Here's how the part is built. I have some questions about the finished solid (model axes, mm). A direction names the side the tool comes from. Coordinates: 2 decimals unless noted, no trailing zeros. Write each loop counter-clockwise with the first axis right and the second up, starting at its lowest first coordinate (ties: lowest second). Pieces come first, ordered by that corner, then holes. Notation, with made-up numbers: (43.5, -33.5) -> (57.5, -33.5) arc R21 cw to (57.5, -26.5) -> close; hole circle Ø3 at (65, -37). An arc over 180 degrees is marked (long way). Put each result on its own line as item: value.
```python
from build123d import *

# Parameters (mm, degrees)
CROQUIS1_R                = 20
SALIENTE_EXTRUIR1_DEPTH   = 45
SALIENTE_EXTRUIR1_2_DEPTH = 45
CROQUIS2_W                = 40
CROQUIS2_H                = 80
SALIENTE_EXTRUIR2_DEPTH   = 45
CORTAR_EXTRUIR2_DEPTH     = 7.6
CROQUIS4_R                = 5.5
CORTAR_EXTRUIR3_DEPTH     = 50
CROQUIS5_W                = 20
CROQUIS5_H                = 40
CORTAR_EXTRUIR4_DEPTH     = 40
CROQUIS6_W                = 20
CROQUIS6_H                = 6.5
CROQUIS6_H_2              = 7
CORTAR_EXTRUIR5_DEPTH     = 12
CORTAR_EXTRUIR6_START     = -27
CROQUIS7_W                = 20
CROQUIS7_H                = 13.910937509
CORTAR_EXTRUIR6_DEPTH     = 12


with BuildPart() as part:
    # Croquis1 → Saliente-Extruir1 (new body)
    with BuildSketch(Plane(origin=(0, 0, 0), x_dir=(0, 1, 0), z_dir=(0, 0, 1))):
        with Locations(Location((-40, 0, 0), (0, 0, 90))):
            Circle(CROQUIS1_R)
    extrude(amount=SALIENTE_EXTRUIR1_DEPTH)



with BuildPart() as body_2:
    # Croquis1 → Saliente-Extruir1 2 (new body)
    with BuildSketch(Plane(origin=(0, 0, 0), x_dir=(0, 1, 0), z_dir=(0, 0, 1))):
        with Locations(Location((40, 0, 0), (0, 0, 90))):
            Circle(CROQUIS1_R)
    extrude(amount=SALIENTE_EXTRUIR1_2_DEPTH)


with BuildPart() as part_1:
    add(part.part)

    add(body_2.part)  # Saliente-Extruir2 merges body 2
    # Croquis2 → Saliente-Extruir2 (add)
    with BuildSketch(Plane.XY.offset(45)):
        Rectangle(CROQUIS2_W, CROQUIS2_H)
    extrude(amount=-SALIENTE_EXTRUIR2_DEPTH)

    # Croquis3 → Cortar-Extruir2 (cut)
    with BuildSketch(Plane.XY.offset(45)):
        with BuildLine():
            Line((-16.5, 42.5), (-4.355962306, 43.357914886))
            Line((-4.355962306, 43.357914886), (-2.5, 56.5))
            ThreePointArc((-2.5, 56.5), (0, 59), (2.5, 56.5))
            Line((2.5, 56.5), (3.889087297, 43.889087297))
            Line((3.889087297, 43.889087297), (16.5, 42.5))
            ThreePointArc((16.5, 42.5), (19, 40), (16.5, 37.5))
            Line((16.5, 37.5), (3.889087297, 36.110912703))
            Line((3.889087297, 36.110912703), (2.5, 23.5))
            ThreePointArc((2.5, 23.5), (0, 21), (-2.5, 23.5))
            Line((-2.5, 23.5), (-3.889087297, 36.110912703))
            Line((-3.889087297, 36.110912703), (-16.5, 37.5))
            ThreePointArc((-16.5, 37.5), (-19, 40), (-16.5, 42.5))
        make_face()
    extrude(amount=-CORTAR_EXTRUIR2_DEPTH, mode=Mode.SUBTRACT)

    # Croquis4 → Cortar-Extruir3 (cut)
    with BuildSketch(Plane.XY.offset(45)):
        with Locations((0, 40)):
            Circle(CROQUIS4_R)
    extrude(amount=-CORTAR_EXTRUIR3_DEPTH, mode=Mode.SUBTRACT)

    # Croquis5 → Cortar-Extruir4 (cut)
    with BuildSketch(Plane(origin=(0, 0, 0), x_dir=(1, 0, 0), z_dir=(0, 0, -1))):
        with Locations((0, 30)):
            Rectangle(CROQUIS5_W, CROQUIS5_H)
    extrude(amount=-CORTAR_EXTRUIR4_DEPTH, mode=Mode.SUBTRACT)

    # Croquis6 → Cortar-Extruir5 (cut)
    with BuildSketch(Plane(origin=(0, 0, 0), x_dir=(1, 0, 0), z_dir=(0, 0, -1))):
        with Locations((0, 53.25)):
            Rectangle(CROQUIS6_W, CROQUIS6_H)
        with Locations((0, 6.5)):
            Rectangle(CROQUIS6_W, CROQUIS6_H_2)
    extrude(amount=-CORTAR_EXTRUIR5_DEPTH, mode=Mode.SUBTRACT)

    # Croquis7 → Cortar-Extruir6 (cut)
    with BuildSketch(Plane(origin=(0, 0, 0), x_dir=(1, 0, 0), z_dir=(0, 0, -1)).offset(CORTAR_EXTRUIR6_START)):
        with Locations((0, 56.955468755)):
            Rectangle(CROQUIS7_W, CROQUIS7_H)
    extrude(amount=-CORTAR_EXTRUIR6_DEPTH, mode=Mode.SUBTRACT)


solid = part_1.part
```
Item 1: Imagine slicing it at C-C on z = 30.5. Write out the boundary of the cut face in (x, y), then the cut area to 3 significant figures.
Output:
outline: (-20, -40) arc R20 ccw to (-10, -57.32) -> (-10, -10) -> (10, -10) -> (10, -57.32) arc R20 ccw to (20, -40) -> (20, 40) arc R20 ccw to (-20, 40) -> close; hole circle Ø11 at (0, 40)
area: 3,380 mm²
Item 2: For P1, Ø10, axis at x = 4.5, y = -33.5, coming from the -Z side; P2, Ø2, axis at x = 3.5, y = -10.5, coming from the -Z side; P3, Ø4, axis at x = 11, z = 16, coming from the +Y side, each with a flat end and sliding along its axis, tell me the tip position at first contact or that it passes through.
Output:
P1: stops at z = 40
P2: stops at z = 12
P3: stops at y = 57.86
Item 3: Imagine slicing it at A-A on x = 0. Write out the boundary of the cut face in (y, z).
Output:
outline: (-60, 0) -> (-56.5, 0) -> (-56.5, 12) -> (-50, 12) -> (-50, 27) -> (-60, 27) -> close; (-60, 39) -> (-50, 39) -> (-50, 40) -> (-10, 40) -> (-10, 12) -> (-3, 12) -> (-3, 0) -> (34.5, 0) -> (34.5, 37.4) -> (21, 37.4) -> (21, 45) -> (-60, 45) -> close; (45.5, 0) -> (60, 0) -> (60, 45) -> (59, 45) -> (59, 37.4) -> (45.5, 37.4) -> close
Item 4: If we mould it in two halves opening along Z, with no side actions, what happens to faces 5 (the flat face through (0, -10, 26)), 6 (the flat face through (-11, 40, 37.4)), 7 (the flat face through (0, 14, 0)), 8 (the flat face through (0, -55, 39))? For each: released by +Z, released by -Z, zero draft, split by the parting line, or undercut.
Output:
face 5: zero draft
face 6: released by +Z
face 7: released by -Z
face 8: undercut
Item 5: Imagine slicing it at B-B on z = 4.5. Write out the boundary of the cut face in (x, y), then the cut area to 3 significant figures.
Output:
outline: (-20, -40) arc R20 ccw to (20, -40) -> (20, 40) arc R20 ccw to (-20, 40) -> close; hole (-10, -56.5) -> (10, -56.5) -> (10, -3) -> (-10, -3) -> close; hole circle Ø11 at (0, 40)
area: 3,290 mm²
Item 6: Please list where these lines run through material, in increasing order: line 1 along Y through (x, z) = (0, 18); line 2 along X through (y, z) = (-31.5, 36.5); line 3 along Y through (x, z) = (-3, 26.5). Write a range as from..to.
Output:
line 1: y = -60..-50, -10..34.5, 45.5..60
line 2: x = -20..-10, 10..20
line 3: y = -59.77..-50, -10..35.39, 44.61..59.77
Item 7: Imagine slicing it at D-D on x = 7. Write out the boundary of the cut face in (y, z) (3 decimals), then the cut area to 3 significant figures.
Output:
outline: (-58.735, 0) -> (-56.5, 0) -> (-56.5, 12) -> (-50, 12) -> (-50, 27) -> (-58.735, 27) -> close; (-58.735, 39) -> (-50, 39) -> (-50, 40) -> (-10, 40) -> (-10, 12) -> (-3, 12) -> (-3, 0) -> (58.735, 0) -> (58.735, 45) -> (43.546, 45) -> (43.546, 37.4) -> (36.454, 37.4) -> (36.454, 45) -> (-58.735, 45) -> close
area: 3,370 mm²
Item 8: Which directions (+Z, -Z, +X, -X, +Y, -Y) give clear straight access to the entire face, cutting with the end or side of a thin tool? Please do faces 1 (the flat face through (-3.44, 49.84, 41.25)), 2 (the flat face through (0, -50, 19)), 3 (the cylindrical face through (-0.716, 45.453, 18.962)), 4 (the flat face through (0, -55, 27)).
Output:
face 1: +Z
face 2: -Z
face 3: +Z, -Z
face 4: -Y
